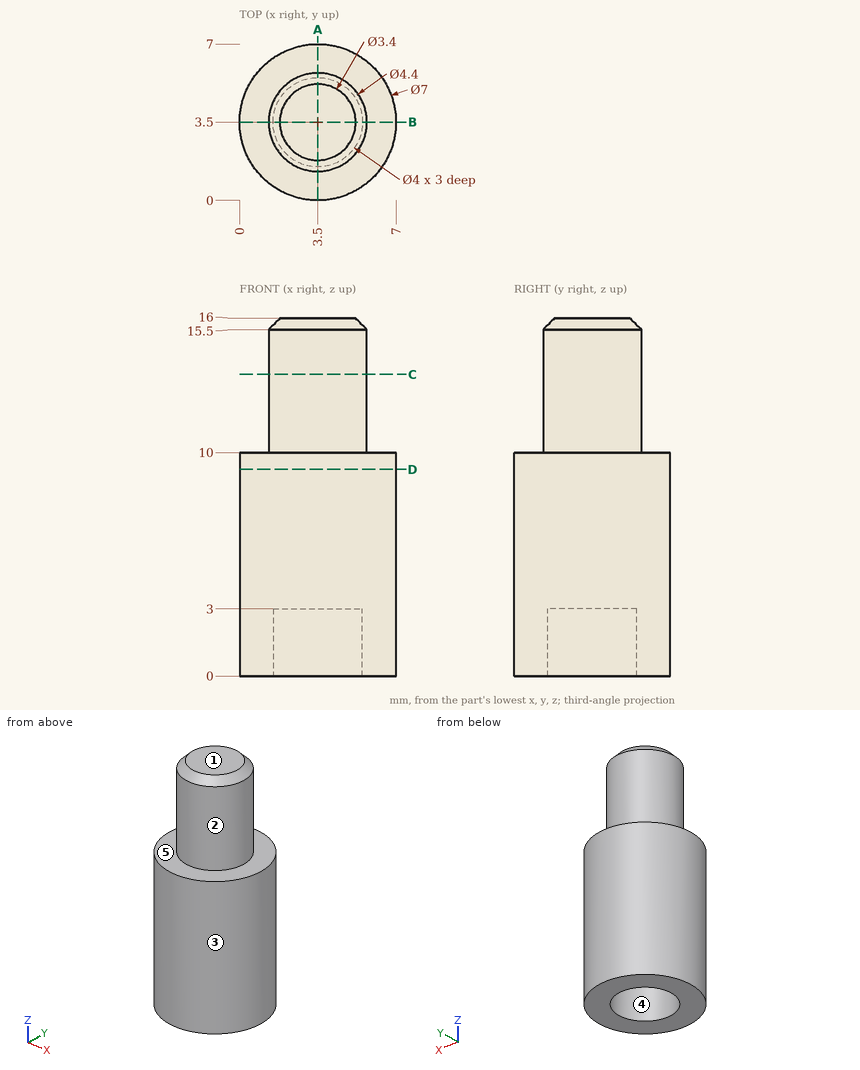
The drawing under review shows one solid part. Ordinate dimensions are in mm from its lowest x, y, z. A direction names the side the tool comes from. Round coordinates to 2 decimals unless told otherwise and drop trailing zeros. Loops run counter-clockwise (first coordinate to the right, second up) from the corner with the lowest first, then second, coordinate; pieces in that order, holes last. Notation, with made-up numbers: (43.25, 24.5) - (52.25, 24.5) arc R17 cw to (52.25, 42.5) - close; hole circle Ø6 at (46, 44). An arc over 180 degrees is marked (long way). One line per question, with ' | ' between items.
Q1. Take a section at A-A (x = 3.5). Give the boundary of the cut face in (y, z).
Taken from the geometry:
outline: (0, 0) - (1.5, 0) - (1.5, 3) - (5.5, 3) - (5.5, 0) - (7, 0) - (7, 10) - (5.7, 10) - (5.7, 15.5) - (5.2, 16) - (1.8, 16) - (1.3, 15.5) - (1.3, 10) - (0, 10) - close
Q2. For line 1 along Y through (x, z) = (3.5, 2.2); line 2 along Z through (x, y) = (1.25, 5); line 3 along Z through (x, y) = (4.25, 5), list the stretches that pass through material, from the lowest coordinate up. Write a range as [from, to].
Taken from the geometry:
line 1: y = [0, 1.5], [5.5, 7] | line 2: z = [0, 10] | line 3: z = [3, 16]
Q3. Take a section at C-C (z = 13.5). Give the boundary of the cut face in (x, y).
Taken from the geometry:
outline: circle Ø4.4 at (3.5, 3.5)
Q4. Take a section at D-D (z = 9.25). Give the boundary of the cut face in (x, y), and give its area (3 significant figures).
Taken from the geometry:
outline: circle Ø7 at (3.5, 3.5) | area: 38.5 mm²
Q5. Tool access review of the marked faces 1 and 2: name each direction out of +Z, -Z, +X, -X, +Y, -Y from which nothing blocks a thin tool from reaching the whole face with its end or side.
Taken from the geometry:
face 1: +Z, +X, -X, +Y, -Y | face 2: +Z
Q6. For pin 1 (3 mm diameter, centred on y = 1.5, z = 12.5, fed in from -X); pin 2 (1.5 mm diameter, centred on y = 1.5, z = 10.5, fed in from -X); pin 3 (2 mm diameter, centred on y = 1.5, z = 5, fed in from -X), all flat-tipped, find the tip position at first contact; note any pin that passes through.
Taken from the geometry:
pin 1: stops at x = 1.36 | pin 2: stops at x = 0.31 | pin 3: stops at x = 0.15
Q7. The part is to be moulded in two halves that separate along X. For the marked faces 3, 4 and 5, say which applies: released by +X, released by -X, zero draft, split by the parting line, or undercut.
Taken from the geometry:
face 3: split by the parting line | face 4: undercut | face 5: zero draft
